from build123d import *

# Parameters (mm, degrees)
SKETCH1_W                        = 19.05
SKETCH1_H                        = 427.342121692
BOSS_EXTRUDE1_DEPTH              = 53
SKETCH2_W                        = 19.05
SKETCH2_H                        = 440.042121692
BOSS_EXTRUDE2_DEPTH              = 56.3
BOSS_EXTRUDE3_DEPTH              = 19.05
F_15_64_0_23438_DIAMETER_HOLE1_D = 5.953252
SKETCH4_R                        = 6.35
CUT_EXTRUDE1_DEPTH               = 20.05
HOLE1_D                          = 3.175
HOLE1_DEPTH                      = 31.75
HOLE1_CSINK_D                    = 10.16
HOLE1_CSINK_ANGLE                = 82
HOLE1_TIP                        = 0.953866233
HOLE_D                           = 3.175
HOLE_DEPTH                       = 31.75
HOLE_CSINK_D                     = 10.16
HOLE_CSINK_ANGLE                 = 82
HOLE_TIP                         = 0.953866233
HOLE3_D                          = 3.175
HOLE3_DEPTH                      = 31.75
HOLE3_CSINK_D                    = 10.16
HOLE3_CSINK_ANGLE                = 82
HOLE3_TIP                        = 0.953866233
HOLE4_D                          = 3.175
HOLE4_DEPTH                      = 31.75
HOLE4_CSINK_D                    = 10.16
HOLE4_CSINK_ANGLE                = 82
HOLE4_TIP                        = 0.953866233
HOLE5_D                          = 3.175
HOLE5_DEPTH                      = 31.75
HOLE5_CSINK_D                    = 10.16
HOLE5_CSINK_ANGLE                = 82
HOLE5_TIP                        = 0.953866233
HOLE6_D                          = 3.175
HOLE6_DEPTH                      = 31.75
HOLE6_CSINK_D                    = 10.16
HOLE6_CSINK_ANGLE                = 82
HOLE6_TIP                        = 0.953866233


with BuildPart() as part:
    # Sketch1 → Boss-Extrude1 (new body)
    with BuildSketch(Plane.XY):
        with Locations((-331.779465963, -213.671060846)):
            Rectangle(SKETCH1_W, SKETCH1_H)
    extrude(amount=BOSS_EXTRUDE1_DEPTH)

    # Sketch2 → Boss-Extrude2 (add)
    with BuildSketch(Plane.XY.offset(53)):
        with Locations((-331.779465963, -207.321060846)):
            Rectangle(SKETCH2_W, SKETCH2_H)
    extrude(amount=BOSS_EXTRUDE2_DEPTH)

    # Sketch3 → Boss-Extrude3 (add, through all)
    with BuildSketch(Plane.ZY.offset(341.304465963)):
        Polygon((0, -427.342121692), (109.3, -427.342121692), (109.3, -464.26606302), (0, -431.185843453), align=None)
    extrude(amount=-BOSS_EXTRUDE3_DEPTH)

    # 15/64 (0.23438) Diameter Hole1 (through all)
    with Locations(Plane.ZY.offset(341.304465963)):
        with Locations((97.748316108, -37.83597394), (97.748316108, -104.51097394), (46.948316108, -71.17347394), (92.682630332, -146.588148739), (96.973742428, -195.635784431), (59.351224796, -174.21579854)):
            Hole(F_15_64_0_23438_DIAMETER_HOLE1_D / 2)

    # Sketch4 → Cut-Extrude1 (cut, through all)
    with BuildSketch(Plane.ZY.offset(341.304465963)):
        with Locations((75.523316108, -71.17347394)):
            Circle(SKETCH4_R)
        with Locations((85.33943188, -171.942125034)):
            Circle(SKETCH4_R)
    extrude(amount=-CUT_EXTRUDE1_DEPTH, mode=Mode.SUBTRACT)

    # Hole1
    with Locations(Plane(origin=(-124.004465969, 10.424290059, 122), x_dir=(-1, 0, 0), z_dir=(0, 0, 1))):
        with Locations((113.649999994, 128.807623392), (113.649999994, 23.940956725), (-94.599999994, 161.374290059), (94.599999994, 161.374290059), (0, 161.374290059), (0, 193.124290059), (0, 440.553783621), (0, 301.970350905), (40.979166666, 301.970350905), (166.795833328, 301.970350905), (207.774999994, 440.553783621), (207.774999994, 333.02141023), (207.774999994, 225.48903684), (207.774999994, 137.424290059), (207.774999994, 10.424290059), (-207.774999994, 10.424290059), (-207.774999994, 137.424290059), (-207.774999994, 225.48903684), (-207.774999994, 333.02141023), (-207.774999994, 440.553783621), (-166.795833328, 301.970350905), (-40.979166666, 301.970350905), (-113.649999994, 23.940956725), (-113.649999994, 128.807623392)):
            CounterSinkHole(HOLE1_D / 2, HOLE1_CSINK_D / 2, depth=HOLE1_DEPTH, counter_sink_angle=HOLE1_CSINK_ANGLE)
            with Locations((0, 0, -(HOLE1_DEPTH + HOLE1_TIP / 2))):  # 118° drill point
                Cone(0, HOLE1_D / 2, HOLE1_TIP, mode=Mode.SUBTRACT)

    # Hole
    with Locations(Plane(origin=(-124.004465969, 25.4, -155.286738577), x_dir=(-1, 0, 0), z_dir=(0, 1, 0))):
        with Locations((113.649999994, 236.436738577), (207.774999994, 236.436738577)):
            CounterSinkHole(HOLE_D / 2, HOLE_CSINK_D / 2, depth=HOLE_DEPTH, counter_sink_angle=HOLE_CSINK_ANGLE)
            with Locations((0, 0, -(HOLE_DEPTH + HOLE_TIP / 2))):  # 118° drill point
                Cone(0, HOLE_D / 2, HOLE_TIP, mode=Mode.SUBTRACT)

    # Hole3
    with Locations(Plane(origin=(-124.004465969, 12.7, -155.286738577), x_dir=(-1, 0, 0), z_dir=(0, 1, 0))):
        with Locations((207.774999994, 172.261738577), (126.349999994, 172.261738577)):
            CounterSinkHole(HOLE3_D / 2, HOLE3_CSINK_D / 2, depth=HOLE3_DEPTH, counter_sink_angle=HOLE3_CSINK_ANGLE)
            with Locations((0, 0, -(HOLE3_DEPTH + HOLE3_TIP / 2))):  # 118° drill point
                Cone(0, HOLE3_D / 2, HOLE3_TIP, mode=Mode.SUBTRACT)

    # Hole4
    with Locations(Plane(origin=(-124.004465969, 10.424290059, -12.7), x_dir=(1, 0, 0), z_dir=(0, 0, -1))):
        with Locations((-207.774999994, 333.02141023), (-207.774999994, 225.48903684), (-207.774999994, 137.424290059), (-172.166666661, 4.074290059), (-146.083333327, 4.074290059), (-94.599999994, 161.374290059), (0, 161.374290059), (94.599999994, 161.374290059), (146.083333327, 4.074290059), (172.166666661, 4.074290059), (207.774999994, 137.424290059), (207.774999994, 225.48903684), (207.774999994, 333.02141023), (166.795833328, 301.970350905), (40.979166666, 301.970350905), (-40.979166666, 301.970350905), (-166.795833328, 301.970350905), (0, 193.124290059), (0, 301.970350905), (0, 412.366411751), (-126.349999994, 106.824290059), (-126.349999994, 58.624290059), (126.349999994, 58.624290059), (126.349999994, 106.824290059)):
            CounterSinkHole(HOLE4_D / 2, HOLE4_CSINK_D / 2, depth=HOLE4_DEPTH, counter_sink_angle=HOLE4_CSINK_ANGLE)
            with Locations((0, 0, -(HOLE4_DEPTH + HOLE4_TIP / 2))):  # 118° drill point
                Cone(0, HOLE4_D / 2, HOLE4_TIP, mode=Mode.SUBTRACT)

    # Hole5
    with Locations(Plane(origin=(-124.004465969, -363.229637966, -268.375064111), x_dir=(1, 0, 0), z_dir=(0, -0.957123977, -0.289678603))):
        with Locations((207.774999994, 613.051808534), (-207.774999994, 613.051808534), (-207.774999994, 456.277103296), (-207.774999994, 769.826513772), (-108.649999997, 456.277103296), (-108.649999997, 630.126513772), (-108.649999997, 769.826513772), (-207.774999994, 362.200879148), (-207.774999994, 305.10273792), (0, 305.10273792), (0, 362.200879148), (207.774999994, 305.10273792), (207.774999994, 362.200879148), (108.649999997, 769.826513772), (108.649999997, 630.126513772), (108.649999997, 456.277103296), (207.774999994, 769.826513772), (207.774999994, 456.277103296)):
            CounterSinkHole(HOLE5_D / 2, HOLE5_CSINK_D / 2, depth=HOLE5_DEPTH, counter_sink_angle=HOLE5_CSINK_ANGLE)
            with Locations((0, 0, -(HOLE5_DEPTH + HOLE5_TIP / 2))):  # 118° drill point
                Cone(0, HOLE5_D / 2, HOLE5_TIP, mode=Mode.SUBTRACT)

    # Hole6
    with Locations(Plane(origin=(-354.004465963, 10.424290059, -155.286738577), x_dir=(0, -0.995945413, 0.089959629), z_dir=(-1, 0, 0))):
        with Locations((637.870011036, 553.595098153), (52.960474704, 241.752641108), (47.697836423, 183.489834462), (434.459074831, 134.806234549), (453.103621196, 177.188747915), (478.414399376, 275.292665941), (488.870508314, 435.756794718), (636.071223534, 609.111420407), (609.449424187, 543.22015483), (559.371199386, 359.303721429), (507.038658285, 229.776136946)):
            CounterSinkHole(HOLE6_D / 2, HOLE6_CSINK_D / 2, depth=HOLE6_DEPTH, counter_sink_angle=HOLE6_CSINK_ANGLE)
            with Locations((0, 0, -(HOLE6_DEPTH + HOLE6_TIP / 2))):  # 118° drill point
                Cone(0, HOLE6_D / 2, HOLE6_TIP, mode=Mode.SUBTRACT)


solid = part.part
Build history of the part. All positions in model axes, mm. A direction names the side the tool comes from. Coordinates: 2 decimals unless noted, no trailing zeros. Write item = value, one per line. Start each with the question number.
1) Two-plate mould, pull along X, no slides. Class faces 3 (the face through (-332.633, -447.14, 86.054)), 4 (the face through (-341.304, -222, 55)), 5 (the face through (-332, 0, 26)): pulls with the +X half, pulls with the -X half, needs draft (parallel to the pull), parting line crosses it, or undercut.
2) Wall check: line 1 along Z through (x, y) = (-340, -71.5); line 2 along Y through (x, z) = (-331, 9.5); line 3 along Y through (x, z) = (-332.75, 7). Give the ranges that are in metal, low to high. Write a range as from..to.
3) Flat gauge pins, fed straight in: pin 1 Ø6 at (x, z) = (-332, 69.5) entering from -Y; pin 2 Ø3 at (x, y) = (-331.78, -322.6) entering from +Z; pin 3 Ø4 at (x, z) = (-329.5, 31) entering from +Y; pin 4 Ø10 at (y, z) = (-71.17, 75.52) entering from +X. Where does each tip first touch, or does it go through?
4) 3-axis set-ups, long thin cutter, end or side, ignore diameter. For faces 1 (the face through (-331.91, -447.96, 55.42)), 2 (the face through (-332, 6, 53)): which of +Z, -Z, +X, -X, +Y, -Y reach the whole face in a straight line?
From the geometry:
q1.face_3 = undercut
q1.face_4 = pulls with the -X half
q1.face_5 = needs draft
q2.line_1 = 0..43.99, 49.91..69.18, 81.86..109.3
q2.line_2 = -434.06..-323.98, -321.21..-216.45, -213.68..-128.38, -125.62..0
q2.line_3 = -433.3..-323.85, -321.34..-216.32, -213.81..-128.26, -125.74..0
q3.pin_1 = -453.13
q3.pin_2 = 90.2
q3.pin_3 = 0
q3.pin_4 = through
q4.face_1 = -Z, +X, -X, -Y
q4.face_2 = -Z, +X, -X, +Y
